```python
from build123d import *

# Parameters (mm, degrees)
BOSS_EXTRUDE1_DEPTH = 5.3
SKETCH2_R           = 4
BOSS_EXTRUDE2_DEPTH = 20
FILLET1_R           = 1


with BuildPart() as part:
    # Sketch1 → Boss-Extrude1 (new body)
    with BuildSketch(Plane(origin=(0, 0, 0), x_dir=(0, 0, -1), z_dir=(1, 0, 0))):
        Polygon((-3.723909236, 6.45), (-7.447818473, 0), (-3.723909236, -6.45), (3.723909236, -6.45), (7.447818473, 0), (3.723909236, 6.45), align=None)
    extrude(amount=BOSS_EXTRUDE1_DEPTH)

    # Sketch2 → Boss-Extrude2 (add)
    with BuildSketch(Plane(origin=(0, 0, 0), x_dir=(0, 0, -1), z_dir=(1, 0, 0))):
        Circle(SKETCH2_R)
    extrude(amount=-BOSS_EXTRUDE2_DEPTH)

    # Fillet1
    fillet1_edges = [part.edges().sort_by_distance(p)[0] for p in [
        (5.3, -3.225, 5.585863854),
        (5.3, -6.45, 0),
        (5.3, -3.225, -5.585863854),
        (5.3, 3.225, -5.585863854),
        (5.3, 6.45, 0),
        (0, 3.225, -5.585863854),
        (0, -3.225, -5.585863854),
        (0, -6.45, 0),
        (0, -3.225, 5.585863854),
        (0, 3.225, 5.585863854),
        (0, 6.45, 0),
        (5.3, 3.225, 5.585863854),
    ]]
    fillet(fillet1_edges, radius=FILLET1_R)


solid = part.part
```
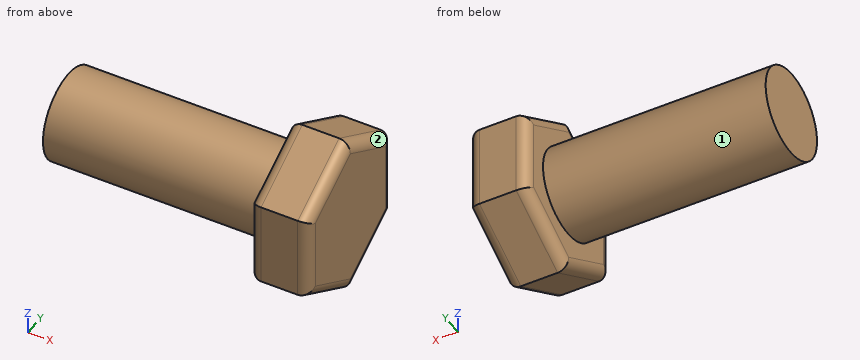
Input: part model. Units: mm. Frame: model coordinates. Face numbers are marked on the shaded views. A direction names the side the tool comes from. Coordinates: 2 decimals unless noted, no trailing zeros. Loops run counter-clockwise (first coordinate to the right, second up) from the corner with the lowest first, then second, coordinate; pieces in that order, holes last.
Q1. Line query: line 1 along X through (y, z) = (2.5, -4.25); line 2 along Y through (x, z) = (-10.5, 3.25); line 3 along Z through (x, y) = (0.5, 1.5). Output: solid intervals per line, ascending.
Results are:
line 1: x = 0 to 5.3
line 2: y = -2.33 to 2.33
line 3: z = -6.43 to 6.43
Q2. Section A-A, the plane z = 0. Return the cut outline in (x, y), and give its area (3 significant figures).
Results are:
outline: (-20, -4) - (0, -4) - (0, -5.45) arc R1 ccw to (1, -6.45) - (4.3, -6.45) arc R1 ccw to (5.3, -5.45) - (5.3, 5.45) arc R1 ccw to (4.3, 6.45) - (1, 6.45) arc R1 ccw to (0, 5.45) - (0, 4) - (-20, 4) - close
area: 228 mm2
Q3. Section B-B, the plane x = 1.5. Return the cut outline in (y, z), and give its area (3 significant figures).
Results are:
outline: (-6.45, -3.72) - (0, -7.45) - (6.45, -3.72) - (6.45, 3.72) - (0, 7.45) - (-6.45, 3.72) - close
area: 144 mm2
Q4. Set-up query: the marked faces 1 and 2. Return all of +Z, -Z, +X, -X, +Y, -Y with unobstructed straight access to the full face (end or side cutting, diameter ignored); none if empty.
Results are:
face 1: -X
face 2: +Z, +X, +Y
Q5. Section C-C, the plane x = -17.5. Return the cut outline in (y, z), and give its area (3 significant figures).
Results are:
outline: circle Ø8 at (0, 0)
area: 50.3 mm2
Q6. Contact query for flat-ended pins moving along their axis: pin 1 (6 mm diameter, centred on x = -11.5, y = -1.5, fed in from -Z); pin 2 (6 mm diameter, centred on x = -6.5, y = 2.5, fed in from +Z); pin 3 (1 mm diameter, centred on x = -8.5, y = 2.5, fed in from -Z). Output: stop coordinate, or through.
Results are:
pin 1: stops at z = -4
pin 2: stops at z = 4
pin 3: stops at z = -3.46
